```python
from build123d import *

# Parameters (mm, degrees)
BARRER_L_MINA1_PROFILE_R   = 20
BARRER_L_MINA1_PROFILE_R_2 = 13
CROQUIS166_R               = 6
CROQUIS166_R_2             = 20
SALIENTE_EXTRUIR2_DEPTH    = 11
CROQUIS167_R               = 39
CROQUIS167_R_2             = 13
SALIENTE_EXTRUIR3_DEPTH    = 8
CROQUIS168_R               = 5
CORTAR_EXTRUIR2_DEPTH      = 15
REDONDEO1_R                = 2.5
REDONDEO2_R                = 2.5


with BuildPart() as part:
    # Barrer-L_mina1: sweep along a path in Croquis8
    with BuildLine(Plane.XY) as barrer_l_mina1_path:
        Line((0, 0), (0, 53))
        ThreePointArc((0, 53), (10.251262658, 77.748737342), (35, 88))
        Line((35, 88), (58, 88))
    # Barrer-L_mina1 profile (on start of the path) → Barrer-L_mina1 (sweep)
    with BuildSketch(Plane.ZX):
        Circle(BARRER_L_MINA1_PROFILE_R)
        Circle(BARRER_L_MINA1_PROFILE_R_2, mode=Mode.SUBTRACT)
    sweep(path=barrer_l_mina1_path.line)

    # Croquis166 → Saliente-Extruir2 (add)
    with BuildSketch(Plane(origin=(58, 0, 0), x_dir=(0, 0, -1), z_dir=(1, 0, 0))):
        with BuildLine():
            Line((-40.336065574, 99.324831744), (-22.950819672, 114.424607403))
            ThreePointArc((-22.950819672, 114.424607403), (0.012124177, 122.9999979), (22.969121399, 114.408700501))
            Line((22.969121399, 114.408700501), (40.855221071, 98.852160917))
            ThreePointArc((40.855221071, 98.852160917), (45.491803378, 88.495813939), (41.549621493, 77.8557472))
            Line((41.549621493, 77.8557472), (23.053076053, 61.664554599))
            ThreePointArc((23.053076053, 61.664554599), (0.067834781, 53.000065737), (-22.950819672, 61.575392597))
            Line((-22.950819672, 61.575392597), (-40.336065574, 76.675168256))
            ThreePointArc((-40.336065574, 76.675168256), (-45.5, 88), (-40.336065574, 99.324831744))
        make_face()
        with Locations((-30.5, 88)):
            Circle(CROQUIS166_R, mode=Mode.SUBTRACT)
        with Locations((30.5, 88)):
            Circle(CROQUIS166_R, mode=Mode.SUBTRACT)
        with Locations((0, 88)):
            Circle(CROQUIS166_R_2, mode=Mode.SUBTRACT)
    extrude(amount=-SALIENTE_EXTRUIR2_DEPTH)

    # Croquis167 → Saliente-Extruir3 (add)
    with BuildSketch(Plane.XZ):
        with Locations(Location((0, 0, 0), (0, 0, 270))):
            Circle(CROQUIS167_R)
        with Locations(Location((0, 0, 0), (0, 0, 180))):
            Circle(CROQUIS167_R_2, mode=Mode.SUBTRACT)
    extrude(amount=-SALIENTE_EXTRUIR3_DEPTH)

    # Croquis168 → Cortar-Extruir2 (cut)
    with BuildSketch(Plane.XZ):
        with Locations(Location((0, 30, 0), (0, 0, 270))):
            Circle(CROQUIS168_R)
        with Locations(Location((0, -30, 0), (0, 0, 270))):
            Circle(CROQUIS168_R)
        with Locations(Location((30, 0, 0), (0, 0, 270))):
            Circle(CROQUIS168_R)
        with Locations(Location((-30, 0, 0), (0, 0, 270))):
            Circle(CROQUIS168_R)
    extrude(amount=-CORTAR_EXTRUIR2_DEPTH, mode=Mode.SUBTRACT)

    # Redondeo1
    redondeo1_edges = [part.edges().sort_by_distance(p)[0] for p in [
        (47, 88, -20),
    ]]
    fillet(redondeo1_edges, radius=REDONDEO1_R)

    # Redondeo2
    redondeo2_edges = [part.edges().sort_by_distance(p)[0] for p in [
        (0, 8, -20),
    ]]
    fillet(redondeo2_edges, radius=REDONDEO2_R)


solid = part.part
```
The listing builds one solid part. Answer for the finished solid, in the listing's coordinates (mm). A direction names the side the tool comes from. Coordinates: 2 decimals unless noted, no trailing zeros. Loops run counter-clockwise (first coordinate to the right, second up) from the corner with the lowest first, then second, coordinate; pieces in that order, holes last. Notation, with made-up numbers: (51.25, 5.5) - (95.25, 5.5) arc R29 cw to (95.25, 30.5) - close; hole circle Ø10 at (32, 85.25). An arc over 180 degrees is marked (long way). Use a Markdown table: item, result. Add a question column.
1) The mould has two halves that part along Y. Classify faces 1 (the flat face through (1, 0, -17)), 2 (the cylindrical face through (52.577, 88.659, -45.486)), 3 (the flat face through (52.577, 106.739, -31.787)), 4 (the cylindrical face through (52.58, 93.95, -29.72)): released by +Y, released by -Y, zero draft, split by the parting line, or undercut.
2) The part is cut by section A-A, the plane x = 49. Give the vertices of the cut face in (y, z).
3) For faces 5 (the cylindrical face through (25.12, 3.94, 1.08)), 6 (the flat face through (-17, 8, -17)), 7 (the flat face through (52.577, 69.873, -32.431)), 8 (the cylindrical face through (53, 53, 0)), determine the directions among +Z, -Z, +X, -X, +Y, -Y from which every point of the face is accessible in a straight line to the end or side of a thin tool.
4) The part is cut by section B-B, the plane z = -28.5. Give the vertices of the cut face in (x, y).
5) Find the intervals of material crossed by line 1 (X direction, y = 3.25, z = 0); line 2 (Y direction, x = 22, z = -8.5); line 3 (Y direction, x = 21, z = -21), in increasing order.
6) The part is cut by section C-C, the plane y = 88. State how many separate pieces and enclosed holes the cut face has, and give its area (3 significant figures).
7) Given pin 1 (3 mm diameter, centred on x = 47, y = 66.5, fed in from +Z); pin 2 (1.5 mm diameter, centred on y = 56, z = -7, fed in from -X); pin 3 (1.5 mm diameter, centred on x = -2, y = 84.5, fed in from -Z), each flat-ended and moving along its own axis, determine where each tip first touches the part or whether it passes through.
Here are the results:
| question | item | result |
|---|---|---|
| 1 | face 1 | released by -Y |
| 1 | face 2 | split by the parting line |
| 1 | face 3 | released by +Y |
| 1 | face 4 | undercut |
| 2 | outline | (61.58, 22.95) arc R35 ccw to (61.66, -23.05) - (77.86, -41.55) arc R15 ccw to (98.85, -40.86) - (114.41, -22.97) arc R35 ccw to (114.42, 22.95) - (99.32, 40.34) arc R15 ccw to (76.68, 40.34) - close; hole circle Ø26 at (88, 0); hole circle Ø12 at (88, -30.5); hole circle Ø12 at (88, 30.5) |
| 3 | face 5 | -Y |
| 3 | face 6 | none |
| 3 | face 7 | -Z, +X, -X, -Y |
| 3 | face 8 | +X, -Y |
| 4 | outline | (-26.62, 0) - (-4.77, 0) - (-4.77, 8) - (-26.62, 8) - close; (4.77, 0) - (26.62, 0) - (26.62, 8) - (4.77, 8) - close; (47, 66.43) - (58, 66.43) - (58, 82.34) - (47, 82.34) - close; (47, 93.66) - (58, 93.66) - (58, 109.6) - (47, 109.6) - close |
| 5 | line 1 | x = -39 to -35, -25 to -13, 13 to 25, 35 to 39 |
| 5 | line 2 | y = 0 to 8, 63.79 to 74.55, 95.91 to 104.49 |
| 5 | line 3 | y = 0 to 8 |
| 6 | separate pieces | 3 |
| 6 | enclosed holes | 0 |
| 6 | area | 1,340 mm^2 |
| 7 | pin 1 | stops at z = 30.35 |
| 7 | pin 2 | stops at x = -18.92 |
| 7 | pin 3 | stops at z = -15.33 |
